from build123d import *

# Parameters (mm, degrees)
EXTRUDE_1_DEPTH     = 3
SKETCH_2_R          = 6.5
CUT_EXTRUDE_1_DEPTH = 47.19523785
CUT_EXTRUDE_3_DEPTH = 3.5
SKETCH_4_3_R        = 6
EXTRUDE_3_DEPTH     = 3
SKETCH_5_R          = 1.5
CUT_EXTRUDE_4_DEPTH = 47.19523785
SKETCH_6_R          = 4.5
EXTRUDE_4_DEPTH     = 3
FILLET_1_R          = 15
SKETCH_8_R          = 2
CUT_EXTRUDE_5_DEPTH = 48.077064479
CUT_EXTRUDE_9_DEPTH = 48.077064479
FILLET_3_R          = 20


with BuildPart() as part:
    # 草图1 → 凸台-拉伸1 (new body)
    with BuildSketch(Plane.XY):
        with BuildLine():
            ThreePointArc((10, 35), (0, 45), (-10, 35))
            Line((-10, 35), (10, 35))
        make_face()
        with BuildLine():
            Line((10, 35), (-10, 35))
            ThreePointArc((-10, 35), (0, 25), (10, 35))
        make_face()
        with BuildLine():
            ThreePointArc((10, 35), (0, 25), (-10, 35))
            Line((-10, 35), (-10, -35))
            Line((-10, -35), (10, -35))
            Line((10, -35), (10, 35))
        make_face()
    extrude(amount=EXTRUDE_1_DEPTH)

    # 草图2 → 切除-拉伸1 (cut, through all)
    with BuildSketch(Plane.XY.offset(3)):
        with Locations((0, 35)):
            Circle(SKETCH_2_R)
    extrude(amount=-CUT_EXTRUDE_1_DEPTH, mode=Mode.SUBTRACT)

    # 草图4 → 切除-拉伸3 (cut)
    with BuildSketch(Plane(origin=(0, 0, 0), x_dir=(-1, 0, 0), z_dir=(0, 0, -1))):
        Polygon((10, 30), (6, -35), (10, -35), align=None)
        Polygon((-10, -35), (-6, -35), (-10, 30), align=None)
    extrude(amount=-CUT_EXTRUDE_3_DEPTH, mode=Mode.SUBTRACT)

    # 草图4<3> → 凸台-拉伸3 (add)
    with BuildSketch(Plane(origin=(0, 0, 0), x_dir=(-1, 0, 0), z_dir=(0, 0, -1))):
        with Locations((0, -35)):
            Circle(SKETCH_4_3_R)
    extrude(amount=-EXTRUDE_3_DEPTH)

    # 草图5 → 切除-拉伸4 (cut, through all)
    with BuildSketch(Plane(origin=(0, 0, 0), x_dir=(-1, 0, 0), z_dir=(0, 0, -1))):
        with Locations((0, -35)):
            Circle(SKETCH_5_R)
    extrude(amount=-CUT_EXTRUDE_4_DEPTH, mode=Mode.SUBTRACT)

    # 草图6 → 凸台-拉伸4 (add)
    with BuildSketch(Plane(origin=(0, 0, 0), x_dir=(-1, 0, 0), z_dir=(0, 0, -1))):
        with Locations((-9, -8)):
            Circle(SKETCH_6_R)
    extrude(amount=-EXTRUDE_4_DEPTH)

    # 圆角1
    fillet_1_edges = [part.edges().sort_by_distance(p)[0] for p in [
        (7.930527209, -3.628932859, 1.5),
        (7.402648929, -12.206954903, 1.5),
    ]]
    fillet(fillet_1_edges, radius=FILLET_1_R)

    # 草图8 → 切除-拉伸5 (cut, through all)
    with BuildSketch(Plane.XY.offset(3)):
        with Locations((9, -8)):
            Circle(SKETCH_8_R)
    extrude(amount=-CUT_EXTRUDE_5_DEPTH, mode=Mode.SUBTRACT)

    # 草图11 → 切除-拉伸9 (cut, through all)
    with BuildSketch(Plane.XY.offset(3)):
        with BuildLine():
            Line((3.090604818, -18.5), (6, -35))
            Line((6, -35), (6.812082422, -21.803660643))
            ThreePointArc((6.812082422, -21.803660643), (7.00895024, -20.135596552), (7.391074134, -18.5))
            Line((7.391074134, -18.5), (3.090604818, -18.5))
        make_face()
    extrude(amount=-CUT_EXTRUDE_9_DEPTH, mode=Mode.SUBTRACT)

    # 圆角3
    # the kernel refuses this fillet: 20 mm, written as the material it adds along each edge
    with BuildSketch(Plane(origin=(3.090604818, -18.5, 3), x_dir=(1, 0, 0), z_dir=(0, 0, -1))) as fillet_3_piece_1:
        with BuildLine():
            CenterArc((21.962966165, 9.382761056), FILLET_3_R, 170, 37.978360215)
            Line((2.266811105, 12.85572461), (1.872888004, 12.925183881))
            Line((1.872888004, 12.925183881), (-0.393923101, 0.069459271))
            Line((-0.393923101, 0.069459271), (0, -0.4))
            ThreePointArc((0, -0.4), (2.150234658, -0.4), (3.947219379, -0.187655221))
            Line((3.947219379, -0.187655221), (4.300469316, 0))
        make_face()
    extrude(amount=3)

    # 草图14 → M3 六角凹锥坑螺钉的锥形沉头孔2 (revolve, cut)
    with BuildSketch(Plane(origin=(0, -35, 0), x_dir=(0, 1, 0), z_dir=(1, 0, 0))):
        Polygon((0, 0), (0, 3), (1.7, 3), (1.7, 1.66), (3.36, 0), align=None)
    revolve(axis=Axis((0, -35, -6.35), (0, 0, 1)), mode=Mode.SUBTRACT)


solid = part.part
Input: part model. Units: mm. Frame: model coordinates. A direction names the side the tool comes from. Give positions to 0.01 mm unless a question says otherwise; leave off trailing zeros. Order: outer loops, then holes, each group sorted by start corner. A loop starts at its lowest first (then second) coordinate and runs counter-clockwise, first axis right, second up. Notation, with made-up numbers: (13, 60.25) - (57, 60.25) arc R37 ccw to (57, 98.25) - close; hole circle Ø6 at (0, -33.5). An arc over 180 degrees is marked (long way). Answer as a JSON object with one key per item and string values. Group by question number.
Q1. First-contact query: pin 1 Ø8 at (x, y) = (-5.5, -23) entering from -Z; pin 2 Ø1 at (x, z) = (5, 2) entering from +Y; pin 3 Ø1 at (y, z) = (-9.5, 1.5) entering from +X; pin 4 Ø1.5 at (y, z) = (-1.5, 0.5) entering from +X. Flat tips, straight axial feed; report the tip coordinate or a pass-through.
Q2. Set-up query: faces 1 (the face through (5.674, -33.152, 1.521)), 2 (the face through (10, 32, 1)), 3 (the face through (0, 45, 1)). Return all of +Z, -Z, +X, -X, +Y, -Y with unobstructed straight access to the full face (end or side cutting, diameter ignored); none if empty.
Q3. Cut plane D-D, the plane x = 4.25. Output: boundary loops of the cut face in (y, z), then the cut area to 3 significant figures.
Q4. Mould query, pull axis X, two halves, no side actions, for faces 4 (the face through (-1, 1, 0)), 5 (the face through (-0.07, -36.7, 2.32)), 6 (the face through (-0.846, 41.445, 1.521)), 7 (the face through (-10, 33, 1)). Classes: pulls with the +X half, pulls with the -X half, needs draft (parallel to the pull), parting line crosses it, or undercut.
Q5. Cut plane A-A, the plane x = 0. Output: boundary loops of the cut face in (y, z), then the cut area to 3 significant figures.
Q6. Cut plane C-C, the plane y = -8. Output: boundary loops of the cut face in (x, z), then the cut area to 3 significant figures.
Q7. Cut plane B-B, the plane z = 1.1. Output: boundary loops of the cut face in (x, y) (3 decimals).
Q8. Line query: probe 1 along Y at (x, z) = (0, 2.65); probe 2 along Y at (x, z) = (-1.5, 2.65); probe 3 along X at (y, z) = (-35, 2.65). Output: solid intervals per line, ascending.
Results:
{
 "1": {"pin 1": "z = 0", "pin 2": "y = 43.93", "pin 3": "x = 13.39", "pin 4": "x = 10.39"},
 "2": {"face 1": "+Z, -Z, +X", "face 2": "+Z, -Z, +X, +Y", "face 3": "+Z, -Z, +Y"},
 "3": {"outline": "(-39.24, 0) - (30.08, 0) - (30.08, 3) - (-39.24, 3) - close; (39.92, 0) - (44.05, 0) - (44.05, 3) - (39.92, 3) - close", "area": "220 mm^2"},
 "4": {"face 4": "needs draft", "face 5": "undercut", "face 6": "undercut", "face 7": "pulls with the -X half"},
 "5": {"outline": "(-41, 0) - (-38.36, 0) - (-36.7, 1.66) - (-36.7, 3) - (-41, 3) - close; (-33.3, 1.66) - (-31.64, 0) - (28.5, 0) - (28.5, 3) - (-33.3, 3) - close; (41.5, 0) - (45, 0) - (45, 3) - (41.5, 3) - close", "area": "206 mm^2"},
 "6": {"outline": "(-7.66, 0) - (7, 0) - (7, 3) - (-7.66, 3) - close; (11, 0) - (13.5, 0) - (13.5, 3) - (11, 3) - close", "area": "51.5 mm^2"},
 "7": {"outline": "(-10, 30) - (-6, -35) arc R6 ccw to (6, -35) - (5.357, -31.356) arc R20 cw to (7.391, -18.5) arc R15 cw to (11.95, -11.398) arc R4.5 ccw to (12.344, -4.989) arc R15 cw to (8.521, 5.968) - (10, 30) - (10, 35) arc R10 ccw to (-10, 35) - close; hole circle Ø13 at (0, 35); hole circle Ø4.52 at (0, -35); hole circle Ø4 at (9, -8)"},
 "8": {"probe 1": "-41 to -36.7, -33.3 to 28.5, 41.5 to 45", "probe 2": "-40.81 to -35.8, -34.2 to 28.68, 41.32 to 44.89", "probe 3": "-6 to -1.7, 1.7 to 6"}
}
